Design review of the part built by this model. Coordinates are the model's own, in mm. Face numbers are marked on the shaded views. A direction names the side the tool comes from. Round coordinates to 2 decimals unless told otherwise and drop trailing zeros. Order: outer loops, then holes, each group sorted by start corner. A loop starts at its lowest first (then second) coordinate and runs counter-clockwise, first axis right, second up. Notation, with made-up numbers: M 80.25,-5.5 L 132.25,-5.5 A13 ccw 132.25,4.5 Z; hole C 42,-9 d5. An arc over 180 degrees is marked long. Use a Markdown table: item, result. Add a question column.
(1) Machinability: for the marked faces 1, 2 and 3, which of the approach directions +Z, -Z, +X, -X, +Y, -Y give a long, thin tool a straight path to every point of the face, cutting with its end or side? Answer none if there is none.
(2) Take a section at D-D (z = 31). Write out the cut boundary in (x, y), then the cut area to 3 significant figures.
(3) To check wall thickness, follow probe 1 along Y at (x, z) = (15, 2); probe 2 along X at (y, z) = (2.5, 17); probe 3 along X at (y, z) = (3, 9). State the ranges of each line that lie inside material, in increasing order. Write a range as from..to.
(4) For pin 1 (1.2 mm diameter, centred on x = 2, z = 27.5, fed in from -Y); pin 2 (12 mm diameter, centred on y = 11, z = 9.5, fed in from +X); pin 3 (15.5 mm diameter, centred on x = 0, z = 10, fed in from -Y); pin 4 (3.5 mm diameter, centred on x = -14.09, y = -7.57, fed in from -Z), all flat-tipped, find the tip position at first contact; note any pin that passes through.
(5) Take a section at A-A (y = 0). Count the separate pieces of the cut face and the enclosed holes in it, then the cut area to 3 significant figures.
(6) The part is to be moulded in two halves that separate along Y. For the marked faces 4, 5 and 6, say which applies: released by +Y, released by -Y, zero draft, split by the parting line, or undercut.
(7) Take a section at B-B (z = 9). Write out the cut boundary in (x, y).
```python
from build123d import *

# Parameters (mm, degrees)
SKETCH_R           = 20
PAD_DEPTH          = 5
PAD001_DEPTH       = 7.5
PAD002_DEPTH       = 4
SKETCH003_R        = 2
POCKET_DEPTH       = 24.001
POCKET001_DEPTH    = 27.501
SKETCH005_R        = 2
POCKET002_DEPTH    = 137.008872
POLARPATTERN_COUNT = 8
FILLET_R           = 2


with BuildPart() as part:
    # Sketch → Pad (new body)
    with BuildSketch(Plane.XY):
        Circle(SKETCH_R)
    extrude(amount=PAD_DEPTH)

    # Sketch001 → Pad001 (join, symmetric)
    with BuildSketch(Plane.XZ):
        with BuildLine():
            Line((9, 17), (9, -0.003877))
            Line((9, -0.003877), (-9, -0.003877))
            Line((-9, -0.003877), (-9, 17))
            ThreePointArc((9, 17), (0, 26), (-9, 17))
        make_face()
    extrude(amount=PAD001_DEPTH, both=True)

    # Sketch002 → Pad002 (join, symmetric)
    with BuildSketch(Plane.YZ):
        with BuildLine():
            Line((-4, 13.8), (-4, 30))
            ThreePointArc((4, 30), (0, 34), (-4, 30))
            Line((4, 30), (4, 13.8))
            Line((4, 13.8), (-4, 13.8))
        make_face()
    extrude(amount=PAD002_DEPTH, both=True)

    # Sketch003 (on Face16 of Pad002) → Pocket (cut, through all)
    with BuildSketch(Plane.YZ.offset(4)):
        with Locations((0, 30)):
            Circle(SKETCH003_R)
    extrude(amount=-POCKET_DEPTH, mode=Mode.SUBTRACT)

    # Sketch004 (on Face11 of Pocket) → Pocket001 (cut, through all)
    with BuildSketch(Plane.XZ.offset(7.5)):
        with BuildLine():
            ThreePointArc((-1.5, 22.809475), (0, 11), (1.5, 22.809475))
            Line((1.5, 39.24), (1.5, 22.809475))
            Line((-1.5, 39.24), (1.5, 39.24))
            Line((-1.5, 22.809475), (-1.5, 39.24))
        make_face()
    extrude(amount=-POCKET001_DEPTH, mode=Mode.SUBTRACT)

    # Sketch005 (on Face3 of Pocket001) → Pocket002 (cut, through all)
    with BuildSketch(Plane.XY.offset(5)):
        with Locations((4.609226, 15.321718)):
            Circle(SKETCH005_R)
    pocket002 = extrude(amount=-POCKET002_DEPTH, mode=Mode.SUBTRACT)

    # PolarPattern: Pocket002 ×8 about axis
    polarpattern_axis = Axis((0, 0, 5), (0, 0, 1))
    for i in range(1, POLARPATTERN_COUNT):
        add(pocket002.rotate(polarpattern_axis, i * 360 / POLARPATTERN_COUNT), mode=Mode.SUBTRACT)

    # Fillet
    fillet_edges = [part.edges().sort_by_distance(p)[0] for p in [
        (6.873864, -7.5, 22.809475),
        (-6.873864, -7.5, 22.809475),
        (6.873864, 7.5, 22.809475),
        (-6.873864, 7.5, 22.809475),
    ]]
    fillet(fillet_edges, radius=FILLET_R)


solid = part.part
```
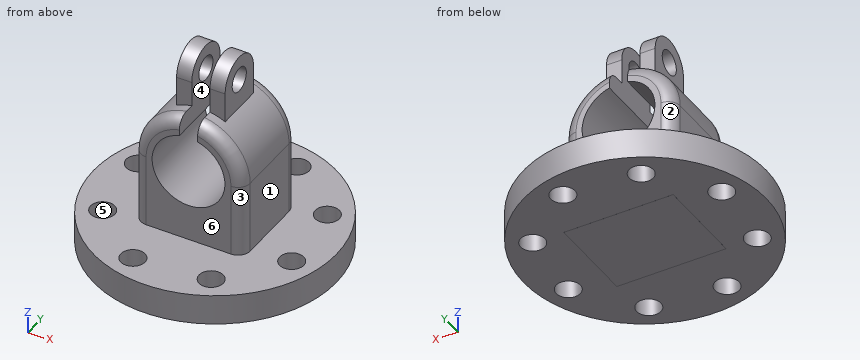
Verdict:
| question | item | result |
|---|---|---|
| 1 | face 1 | +Z, +X, +Y, -Y |
| 1 | face 2 | +Z, -X, +Y |
| 1 | face 3 | +Z, +X, -Y |
| 2 | outline | M -4,-3.87 L -1.5,-3.87 L -1.5,-1.73 L -4,-1.73 Z; M -4,1.73 L -1.5,1.73 L -1.5,3.87 L -4,3.87 Z; M 1.5,-3.87 L 4,-3.87 L 4,-1.73 L 1.5,-1.73 Z; M 1.5,1.73 L 4,1.73 L 4,3.87 L 1.5,3.87 Z |
| 2 | area | 21.4 mm^2 |
| 3 | probe 1 | y = -13.23..-6.58, -2.64..5.79, 9.36..13.23 |
| 3 | probe 2 | x = -9..-6, 6..9 |
| 3 | probe 3 | x = -9..9 |
| 4 | pin 1 | stops at y = -4 |
| 4 | pin 2 | stops at x = 18.72 |
| 4 | pin 3 | stops at y = -20 |
| 4 | pin 4 | passes through |
| 5 | separate pieces | 3 |
| 5 | enclosed holes | 0 |
| 5 | area | 443 mm^2 |
| 6 | face 4 | zero draft |
| 6 | face 5 | undercut |
| 6 | face 6 | released by -Y |
| 7 | outline | M -9,-5.5 A2 ccw -7,-7.5 L 7,-7.5 A2 ccw 9,-5.5 L 9,5.5 A2 ccw 7,7.5 L -7,7.5 A2 ccw -9,5.5 Z |
